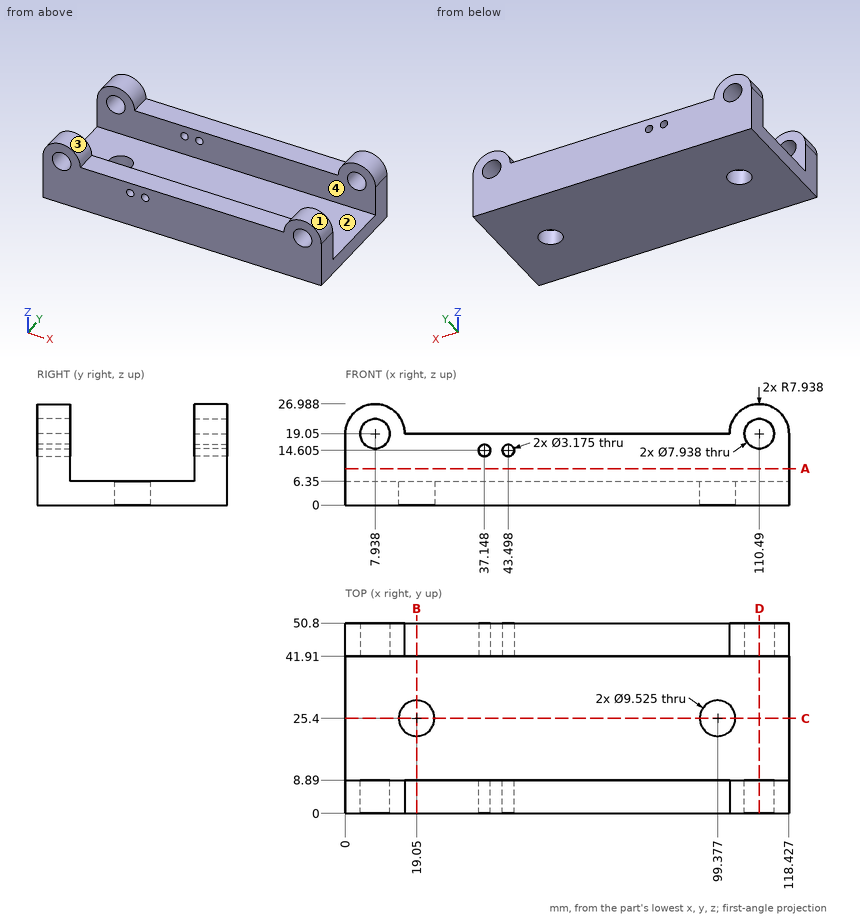
For this review, use the dimensioned drawing (mm, ordinates from the lowest corner) and the shaded views. A direction names the side the tool comes from. Coordinates: 2 decimals unless noted, no trailing zeros. Loops run counter-clockwise (first coordinate to the right, second up) from the corner with the lowest first, then second, coordinate; pieces in that order, holes last. Notation, with made-up numbers: (0, -12.5) - (14, -12.5) arc R27 ccw to (14, 3.5) - close; hole circle Ø2 at (18.5, 68). An arc over 180 degrees is marked (long way). Use one line per item in the form item = value. Start each with the question number.
1) Draft analysis for pull direction X (two halves, no side actions). For the marked faces 1 and 2, state which applies: released by +X, released by -X, zero draft, split by the parting line, or undercut.
2) For the marked faces 3 and 4, list the 3-axis set-ups (+Z, -Z, +X, -X, +Y, -Y) from which the entire face can be reached by the end or side of a thin tool; tool diameter is ignored.
3) Take a section at A-A (z = 9.75). State the section outline as (x, y) points, plus the area to 3 significant figures.
4) Take a section at D-D (x = 110.49). State the section outline as (y, z) points.
5) To check wall thickness, follow probe 1 along X at (y, z) = (25.4, 3) (1 decimal); probe 2 along Y at (x, z) = (70, 14); probe 3 along Z at (x, y) = (110.49, 45.75). State the ranges of each line that lie inside material, in increasing order. Write a range as from..to.
6) For pin 1 (8 mm diameter, centred on x = 74.5, z = 24, fed in from -Y); pin 2 (2 mm diameter, centred on x = 36.5, y = 28.5, fed in from +Z); pin 3 (7 mm diameter, centred on x = 44.5, y = 48.5, fed in from +Z), all flat-tipped, find the tip position at first contact; note any pin that passes through.
7) Take a section at C-C (y = 25.4). State how many separate pieces and enclosed holes the cut face has, plus the area to 3 significant figures.
8) Take a section at B-B (x = 19.05). State the section outline as (y, z) points, plus the area to 3 significant figures.
From the geometry:
q1.face_1 = undercut
q1.face_2 = zero draft
q2.face_3 = +Z, +Y, -Y
q2.face_4 = +Z, +X, -X
q3.outline = (0, 0) - (118.43, 0) - (118.43, 8.89) - (0, 8.89) - close; (0, 41.91) - (118.43, 41.91) - (118.43, 50.8) - (0, 50.8) - close
q3.area = 2,110 mm2
q4.outline = (0, 0) - (50.8, 0) - (50.8, 15.08) - (41.91, 15.08) - (41.91, 6.35) - (8.89, 6.35) - (8.89, 15.08) - (0, 15.08) - close; (0, 23.02) - (8.89, 23.02) - (8.89, 26.99) - (0, 26.99) - close; (41.91, 23.02) - (50.8, 23.02) - (50.8, 26.99) - (41.91, 26.99) - close
q5.probe_1 = 0..14.3, 23.8..94.6, 104.1..118.4
q5.probe_2 = 0..8.89, 41.91..50.8
q5.probe_3 = 0..15.08, 23.02..26.99
q6.pin_1 = through
q6.pin_2 = 6.35
q6.pin_3 = 19.05
q7.separate_pieces = 3
q7.enclosed_holes = 0
q7.area = 631 mm2
q8.outline = (0, 0) - (20.64, 0) - (20.64, 6.35) - (8.89, 6.35) - (8.89, 19.05) - (0, 19.05) - close; (30.16, 0) - (50.8, 0) - (50.8, 19.05) - (41.91, 19.05) - (41.91, 6.35) - (30.16, 6.35) - close
q8.area = 488 mm2
